CAD build for the part. Positions are in the model's coordinates, mm. Face numbers are marked on the shaded views. A direction names the side the tool comes from. Round coordinates to 2 decimals unless told otherwise and drop trailing zeros. Write each loop counter-clockwise with the first axis right and the second up, starting at its lowest first coordinate (ties: lowest second). Pieces come first, ordered by that corner, then holes. Notation, with made-up numbers: (54.25, 7) - (86.25, 7) arc R21 cw to (86.25, 28) - close; hole circle Ø4 at (20.25, -34). An arc over 180 degrees is marked (long way). Put each result on its own line as item: value. Start each with the question number.
Item 1: Drill centre lines: line 1 (Z direction, x = -25.4, y = -3); line 2 (X direction, y = -0.2, z = 0); line 3 (Z direction, x = 25, y = -12). Where is each one in solid material? Low to high. Write a range as from..to.
Item 2: 3-axis set-ups, long thin cutter, end or side, ignore diameter. For the marked faces 4 and 5: which of +Z, -Z, +X, -X, +Y, -Y reach the whole face in a straight line?
Item 3: Mould opens along Z. For the marked faces 1, 2 and 3 say: released by +Z, released by -Z, zero draft, split by the parting line, or undercut.
Item 4: Cut at B-B (z = 25.4). Give the cut face in (x, y), and give its area (3 significant figures).
Item 5: Cut at A-A (x = -25.4). Give the cut face in (y, z), and give its area (3 significant figures).
Item 6: Pin check, flat tips, straight feed: pin 1 Ø6 at (x, y) = (-65.5, -9.5) entering from +Z; pin 2 Ø3 at (x, y) = (62.5, -3) entering from +Z; pin 3 Ø7.5 at (x, z) = (-2, -38.5) entering from +Y. Stop position of each tip, or through.
Item 7: Cut at C-C (y = -4.25). Count the separate pieces of the cut face and the enclosed holes in it, and give its area (3 significant figures).
Item 8: Cut at D-D (z = 0). Give the cut face in (x, y), and give its area (3 significant figures).
```python
from build123d import *

# Parameters (mm, degrees)
SKETCH1_R                                        = 85
BOSS_EXTRUDE1_DEPTH                              = 13
SKETCH2_R                                        = 75.75
CUT_EXTRUDE1_DEPTH                               = 0.5
CBORE_FOR_1_4_SOCKET_HEAD_CAP_SCREW1_D           = 6.7564
CBORE_FOR_1_4_SOCKET_HEAD_CAP_SCREW1_DEPTH       = 15
CBORE_FOR_1_4_SOCKET_HEAD_CAP_SCREW1_CBORE_D     = 11.1125
CBORE_FOR_1_4_SOCKET_HEAD_CAP_SCREW1_CBORE_DEPTH = 7.349998
CBORE_FOR_1_4_SOCKET_HEAD_CAP_SCREW1_TIP         = 2.029827343
F_8_32_TAPPED_HOLE1_D                            = 3.4544
F_8_32_TAPPED_HOLE1_DEPTH                        = 8
F_8_32_TAPPED_HOLE1_TIP                          = 1.037806461
SKETCH9_W                                        = 25.4
SKETCH9_H                                        = 25
WAFER_TWEEZER_SLOT_DEPTH                         = 1
FILLET1_R                                        = 5
SKETCH10_R                                       = 7.5
CUT_EXTRUDE2_DEPTH                               = 0.5
F_8_32_TAPPED_HOLE2_D                            = 3.4544
F_8_32_TAPPED_HOLE2_DEPTH                        = 8
F_8_32_TAPPED_HOLE2_TIP                          = 1.037806461


with BuildPart() as part:
    # Sketch1 → Boss-Extrude1 (new body)
    with BuildSketch(Plane(origin=(0, 0, 0), x_dir=(1, 0, 0), z_dir=(0, 1, 0))):
        with Locations(Location((0, 0, 0), (0, 0, 270))):
            Circle(SKETCH1_R)
    extrude(amount=-BOSS_EXTRUDE1_DEPTH)

    # Sketch2 → Cut-Extrude1 (cut)
    with BuildSketch(Plane(origin=(0, 0, 0), x_dir=(1, 0, 0), z_dir=(0, 1, 0))):
        with Locations(Location((0, 0, 0), (0, 0, 270))):
            Circle(SKETCH2_R)
    extrude(amount=-CUT_EXTRUDE1_DEPTH, mode=Mode.SUBTRACT)

    # CBORE for 1/4 Socket Head Cap Screw1
    with Locations(Plane(origin=(0, -0.5, 0), x_dir=(-1, 0, 0), z_dir=(0, 1, 0))):
        with Locations((25.4, 25.4), (-25.4, 25.4), (-25.4, -25.4), (25.4, -25.4)):
            CounterBoreHole(CBORE_FOR_1_4_SOCKET_HEAD_CAP_SCREW1_D / 2, CBORE_FOR_1_4_SOCKET_HEAD_CAP_SCREW1_CBORE_D / 2, CBORE_FOR_1_4_SOCKET_HEAD_CAP_SCREW1_CBORE_DEPTH, depth=CBORE_FOR_1_4_SOCKET_HEAD_CAP_SCREW1_DEPTH)
            with Locations((0, 0, -(CBORE_FOR_1_4_SOCKET_HEAD_CAP_SCREW1_DEPTH + CBORE_FOR_1_4_SOCKET_HEAD_CAP_SCREW1_TIP / 2))):  # 118° drill point
                Cone(0, CBORE_FOR_1_4_SOCKET_HEAD_CAP_SCREW1_D / 2, CBORE_FOR_1_4_SOCKET_HEAD_CAP_SCREW1_TIP, mode=Mode.SUBTRACT)

    # #8-32 Tapped Hole1
    with Locations(Plane(origin=(0, 0, 0), x_dir=(1, 0, 0), z_dir=(0, 1, 0))):
        with Locations((0, 79), (0, -79)):
            Hole(F_8_32_TAPPED_HOLE1_D / 2, depth=F_8_32_TAPPED_HOLE1_DEPTH)
            with Locations((0, 0, -(F_8_32_TAPPED_HOLE1_DEPTH + F_8_32_TAPPED_HOLE1_TIP / 2))):  # 118° drill point
                Cone(0, F_8_32_TAPPED_HOLE1_D / 2, F_8_32_TAPPED_HOLE1_TIP, mode=Mode.SUBTRACT)

    # Sketch9 → wafer_tweezer_slot (cut)
    with BuildSketch(Plane(origin=(0, 0, 0), x_dir=(1, 0, 0), z_dir=(0, 1, 0))):
        with Locations((63.5, 0)):
            Rectangle(SKETCH9_W, SKETCH9_H)
    extrude(amount=-WAFER_TWEEZER_SLOT_DEPTH, mode=Mode.SUBTRACT)

    # Fillet1
    # the kernel refuses this fillet: 5 mm, written as the material it adds along each edge
    with BuildSketch(Plane(origin=(76.2, 0, -12.5), x_dir=(0, 0, 1), z_dir=(0, -1, 0))) as fillet1_piece_1_section:
        with BuildLine():
            CenterArc((FILLET1_R, FILLET1_R), FILLET1_R, 180, 90)
            Line((0, FILLET1_R), (0, 0))
            Line((0, 0), (FILLET1_R, 0))
        make_face()
    fillet1_piece_1 = extrude(amount=1, mode=Mode.PRIVATE)
    fillet1_piece_1 = fillet1_piece_1 - Plane(origin=(0, -0.25, 0), x_dir=(0, 0, 1), z_dir=(0, 1, 0)) * Cylinder(75.75, 23, mode=Mode.PRIVATE)
    add(fillet1_piece_1)
    with BuildSketch(Plane(origin=(76.2, 12.5, -12.5), x_dir=(0, 0, 1), z_dir=(0, -1, 0))) as fillet1_piece_2_section:
        with BuildLine():
            CenterArc((FILLET1_R, FILLET1_R), FILLET1_R, 180, 90)
            Line((0, FILLET1_R), (0, 0))
            Line((0, 0), (FILLET1_R, 0))
        make_face()
    fillet1_piece_2 = extrude(amount=13.5, mode=Mode.PRIVATE)
    fillet1_piece_2 = split(fillet1_piece_2, bisect_by=Plane(origin=(73.966184718, -0.5, -12.010793602), z_dir=(0, -1, 0)), keep=Keep.TOP, mode=Mode.PRIVATE)
    add(fillet1_piece_2)
    with BuildSketch(Plane(origin=(76.2, 0, 12.5), x_dir=(0, 0, -1), z_dir=(0, -1, 0))) as fillet1_piece_3_section:
        with BuildLine():
            CenterArc((FILLET1_R, -FILLET1_R), FILLET1_R, 90, 90)
            Line((0, -FILLET1_R), (0, 0))
            Line((0, 0), (FILLET1_R, 0))
        make_face()
    fillet1_piece_3 = extrude(amount=1, mode=Mode.PRIVATE)
    fillet1_piece_3 = fillet1_piece_3 - Plane(origin=(0, -0.25, 0), x_dir=(0, 0, 1), z_dir=(0, 1, 0)) * Cylinder(75.75, 22, mode=Mode.PRIVATE)
    add(fillet1_piece_3)
    with BuildSketch(Plane(origin=(76.2, 12.5, 12.5), x_dir=(0, 0, -1), z_dir=(0, -1, 0))) as fillet1_piece_4_section:
        with BuildLine():
            CenterArc((FILLET1_R, -FILLET1_R), FILLET1_R, 90, 90)
            Line((0, -FILLET1_R), (0, 0))
            Line((0, 0), (FILLET1_R, 0))
        make_face()
    fillet1_piece_4 = extrude(amount=13.5, mode=Mode.PRIVATE)
    fillet1_piece_4 = split(fillet1_piece_4, bisect_by=Plane(origin=(73.966184718, -0.5, 12.010793602), z_dir=(0, -1, 0)), keep=Keep.TOP, mode=Mode.PRIVATE)
    add(fillet1_piece_4)
    with BuildSketch(Plane(origin=(50.8, -0.5, 12.5), x_dir=(0, 0, -1), z_dir=(0, -1, 0))) as fillet1_piece_5:
        with BuildLine():
            CenterArc((FILLET1_R, FILLET1_R), FILLET1_R, 180, 90)
            Line((0, FILLET1_R), (0, 0))
            Line((0, 0), (FILLET1_R, 0))
        make_face()
    extrude(amount=0.5)
    with BuildSketch(Plane(origin=(50.8, -0.5, -12.5), x_dir=(0, 0, 1), z_dir=(0, -1, 0))) as fillet1_piece_6:
        with BuildLine():
            CenterArc((FILLET1_R, -FILLET1_R), FILLET1_R, 90, 90)
            Line((0, -FILLET1_R), (0, 0))
            Line((0, 0), (FILLET1_R, 0))
        make_face()
    extrude(amount=0.5)

    # Sketch10 → Cut-Extrude2 (cut)
    with BuildSketch(Plane(origin=(0, -0.5, 0), x_dir=(1, 0, 0), z_dir=(0, 1, 0))):
        with Locations(Location((0, -42.164, 0), (0, 0, 270))):
            Circle(SKETCH10_R)
        with Locations(Location((0, 42.164, 0), (0, 0, 270))):
            Circle(SKETCH10_R)
    extrude(amount=-CUT_EXTRUDE2_DEPTH, mode=Mode.SUBTRACT)

    # #8-32 Tapped Hole2
    with Locations(Plane(origin=(0, -1, 0), x_dir=(1, 0, 0), z_dir=(0, 1, 0))):
        with Locations((0, 42.164), (0, -42.164)):
            Hole(F_8_32_TAPPED_HOLE2_D / 2, depth=F_8_32_TAPPED_HOLE2_DEPTH)
            with Locations((0, 0, -(F_8_32_TAPPED_HOLE2_DEPTH + F_8_32_TAPPED_HOLE2_TIP / 2))):  # 118° drill point
                Cone(0, F_8_32_TAPPED_HOLE2_D / 2, F_8_32_TAPPED_HOLE2_TIP, mode=Mode.SUBTRACT)


solid = part.part
```
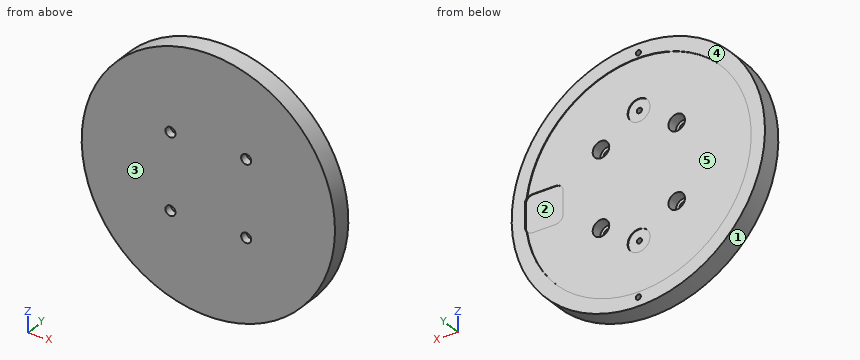
Output values:
1. line 1: -81.12..-30.96, -19.84..19.84, 30.96..81.12
1. line 2: -85..-75.75, 76.2..85
1. line 3: -81.24..-28.75, -22.05..22.05, 28.75..81.24
2. face 4: +Z, -Z, +X, -X, +Y
2. face 5: +Y
3. face 1: split by the parting line
3. face 2: undercut
3. face 3: zero draft
4. outline: (-81.12, -13) - (-28.78, -13) - (-28.78, -7.85) - (-30.96, -7.85) - (-30.96, -0.5) - (-71.36, -0.5) - (-71.36, 0) - (-81.12, 0) - close; (-22.02, -13) - (22.02, -13) - (22.02, -7.85) - (19.84, -7.85) - (19.84, -0.5) - (-19.84, -0.5) - (-19.84, -7.85) - (-22.02, -7.85) - close; (28.78, -13) - (81.12, -13) - (81.12, 0) - (71.36, 0) - (71.36, -0.5) - (30.96, -0.5) - (30.96, -7.85) - (28.78, -7.85) - close
4. area: 1,800 mm2
5. outline: (-13, -81.12) - (0, -81.12) - (0, -71.36) - (-0.5, -71.36) - (-0.5, -30.96) - (-7.85, -30.96) - (-7.85, -28.78) - (-13, -28.78) - close; (-13, -22.02) - (-7.85, -22.02) - (-7.85, -19.84) - (-0.5, -19.84) - (-0.5, 19.84) - (-7.85, 19.84) - (-7.85, 22.02) - (-13, 22.02) - close; (-13, 28.78) - (-7.85, 28.78) - (-7.85, 30.96) - (-0.5, 30.96) - (-0.5, 71.36) - (0, 71.36) - (0, 81.12) - (-13, 81.12) - close
5. area: 1,800 mm2
6. pin 1: z = 57.61
6. pin 2: z = 59.19
6. pin 3: y = -0.5
7. separate pieces: 1
7. enclosed holes: 8
7. area: 22,300 mm2
8. outline: (-85, -13) - (85, -13) - (85, 0) - (76.2, 0) - (76.2, -1) - (50.8, -1) - (50.8, -0.5) - (-75.75, -0.5) - (-75.75, 0) - (-85, 0) - close
8. area: 2,120 mm2
